from build123d import *

# Parameters (mm, degrees)
SKETCH1_W           = 57.15
SKETCH1_H           = 60.325
SKETCH1_W_2         = 6.35
SKETCH1_H_2         = 3.175
SKETCH1_W_3         = 3.175
SKETCH1_H_3         = 6.35
BOSS_EXTRUDE1_DEPTH = 3.175


with BuildPart() as part:
    # Sketch1 → Boss-Extrude1 (new body)
    with BuildSketch(Plane(origin=(0, 0, 0), x_dir=(1, 0, 0), z_dir=(0, 1, 0))):
        with Locations((28.575, 30.1625)):
            Rectangle(SKETCH1_W, SKETCH1_H)
        with Locations((44.45, 30.1625)):
            Rectangle(SKETCH1_W_2, SKETCH1_H_2, mode=Mode.SUBTRACT)
        with Locations((52.3875, 36.5125)):
            Rectangle(SKETCH1_W_3, SKETCH1_H_3, mode=Mode.SUBTRACT)
        with Locations((52.3875, 23.8125)):
            Rectangle(SKETCH1_W_3, SKETCH1_H_3, mode=Mode.SUBTRACT)
        with Locations((52.3875, 49.2125)):
            Rectangle(SKETCH1_W_3, SKETCH1_H_3, mode=Mode.SUBTRACT)
        with Locations((52.3875, 11.1125)):
            Rectangle(SKETCH1_W_3, SKETCH1_H_3, mode=Mode.SUBTRACT)
        with Locations((11.2125, 11.1125)):
            Rectangle(SKETCH1_W_3, SKETCH1_H_3, mode=Mode.SUBTRACT)
        with Locations((11.2125, 49.2125)):
            Rectangle(SKETCH1_W_3, SKETCH1_H_3, mode=Mode.SUBTRACT)
        with Locations((11.2125, 36.5125)):
            Rectangle(SKETCH1_W_3, SKETCH1_H_3, mode=Mode.SUBTRACT)
        with Locations((11.2125, 23.8125)):
            Rectangle(SKETCH1_W_3, SKETCH1_H_3, mode=Mode.SUBTRACT)
        with Locations((31.75, 30.1625)):
            Rectangle(SKETCH1_W_2, SKETCH1_H_2, mode=Mode.SUBTRACT)
        with Locations((19.05, 30.1625)):
            Rectangle(SKETCH1_W_2, SKETCH1_H_2, mode=Mode.SUBTRACT)
        with Locations((6.35, 30.1625)):
            Rectangle(SKETCH1_W_2, SKETCH1_H_2, mode=Mode.SUBTRACT)
    extrude(amount=BOSS_EXTRUDE1_DEPTH)


solid = part.part
Geometry check sheet. Reference: the model listing, model coordinates, mm. Give positions to 0.01 mm unless a question says otherwise; leave off trailing zeros. Order: outer loops, then holes, each group sorted by start corner. A loop starts at its lowest first (then second) coordinate and runs counter-clockwise, first axis right, second up. Notation, with made-up numbers: (8.25, 25) - (44.25, 25) arc R33 cw to (44.25, 61) - close; hole circle Ø4 at (36.5, 32.5). An arc over 180 degrees is marked (long way). Answer as a JSON object with one key per item and string values.
(1) Cross-section at B-B (z = -24.5). Record the cut outline in (x, y) (3 decimals).
Report:
{"outline": "(0, 0) - (9.625, 0) - (9.625, 3.175) - (0, 3.175) - close; (12.8, 0) - (50.8, 0) - (50.8, 3.175) - (12.8, 3.175) - close; (53.975, 0) - (57.15, 0) - (57.15, 3.175) - (53.975, 3.175) - close"}
(2) Draft check along X on faces 1 (the flat face through (28, 3.175, -31)), 2 (the flat face through (3.175, 2, -30)), 3 (the flat face through (57.15, 2, -30)), 4 (the flat face through (32, 2, -31.75)). Enter one of: released by +X, released by -X, zero draft, split by the parting line, or undercut.
Report:
{"face 1": "zero draft", "face 2": "undercut", "face 3": "released by +X", "face 4": "undercut"}
(3) Material ranges on line 1 (Z direction, x = 51, y = 1.7) (1 decimal); line 2 (X direction, y = 2.25, z = -34.5) (3 decimals); line 3 (X direction, y = 2.55, z = -29) (3 decimals), recorded low to high.
Report:
{"line 1": "-60.3 to -52.4, -46 to -39.7, -33.3 to -27, -20.6 to -14.3, -7.9 to 0", "line 2": "0 to 9.625, 12.8 to 50.8, 53.975 to 57.15", "line 3": "0 to 3.175, 9.525 to 15.875, 22.225 to 28.575, 34.925 to 41.275, 47.625 to 57.15"}
(4) Cross-section at C-C (y = 2.3). State how many separate pieces and enclosed holes the cut face has, then the cut area to 3 significant figures.
Report:
{"separate pieces": "1", "enclosed holes": "12", "area": "3,210 mm^2"}
(5) Cross-section at A-A (x = 7). Record the cut outline in (y, z) (3 decimals).
Report:
{"outline": "(0, -60.325) - (3.175, -60.325) - (3.175, -31.75) - (0, -31.75) - close; (0, -28.575) - (3.175, -28.575) - (3.175, 0) - (0, 0) - close"}
